from build123d import *

# Parameters (mm, degrees)
F0_W     = 53
F0_H     = 93
F1_DEPTH = 1
F2_W     = 53
F2_H     = 93
F3_DEPTH = 10
F5_DEPTH = 70
F6_W     = 6
F6_H     = 95.9582039332
F6_H_2   = 4.0417960668
F7_DEPTH = 9
F8_DEPTH = 60


with BuildPart() as f1:
    # F0 (on Top) → F1 (new body)
    with BuildSketch(Plane.XY):
        with Locations((-26.5, 46.5)):
            Rectangle(F0_W, F0_H)
    extrude(amount=F1_DEPTH)

    # F2 (on face) → F3 (join)
    with BuildSketch(Plane.XY.offset(1)):
        with Locations((-26.5, 46.5)):
            Rectangle(F2_W, F2_H)
    extrude(amount=-F3_DEPTH)

    # F4 (on face) → F5 (cut)
    with BuildSketch(Plane.YZ):
        Polygon((93, -9), (92.4582039325, -9), (79.0417960675, -9), (78.4996898418, -9), (77.9999999123, -9), (77.4582039325, -9), (64.0417960675, -9), (63.4996898418, -9), (62.9999999123, -9), (62.4582039325, -9), (49.0417960675, -9), (48.4996898418, -9), (47.9999999123, -9), (47.4582039325, -9), (34.0417960675, -9), (33.4996898418, -9), (32.9999999123, -9), (32.4582039318, -9), (19.0417960668, -9), (18.4996898418, -9), (17.9999999123, -9), (17.4582039318, -9), (4.0417960668, -9), (0, -9), (0, -7.7468557283), (-7.4705565355, -7.7468557283), (-7.4705565355, -22.4550403655), (98.083905875, -22.4550403655), (98.083905875, -6.994248211), (93, -6.994248211), align=None)
        with BuildLine():
            Line((79.0417960675, -9), (92.4582039325, -9))
            ThreePointArc((92.4582039325, -9), (92.6770814653, -8.0077412234), (92.7499976369, -6.994248211))
            ThreePointArc((92.7499976369, -6.994248211), (84.7365672438, -0.0737489182), (79.0417960675, -9))
        make_face()
        with BuildLine():
            Line((64.0417960675, -9), (77.4582039325, -9))
            ThreePointArc((77.4582039325, -9), (71.760587075, -0.0733331419), (63.75, -7))
            ThreePointArc((63.75, -7), (63.8233331419, -8.010587075), (64.0417960675, -9))
        make_face()
        with BuildLine():
            Line((34.0417960675, -9), (47.4582039325, -9))
            ThreePointArc((47.4582039325, -9), (40.75, 0), (34.0417960675, -9))
        make_face()
        with BuildLine():
            ThreePointArc((62.4582039325, -9), (62.6766668581, -8.010587075), (62.75, -7))
            ThreePointArc((62.75, -7), (54.739412925, -0.0733331419), (49.0417960675, -9))
            Line((49.0417960675, -9), (62.4582039325, -9))
        make_face()
        with BuildLine():
            ThreePointArc((32.4582039318, -9), (25.7499999993, 0), (19.0417960668, -9))
            Line((19.0417960668, -9), (32.4582039318, -9))
        make_face()
        with BuildLine():
            ThreePointArc((17.4582039318, -9), (11.3890997117, -0.0292359416), (3.7899564275, -7.7468557283))
            ThreePointArc((3.7899564275, -7.7468557283), (3.8872133859, -8.3791881304), (4.0417960668, -9))
            Line((4.0417960668, -9), (17.4582039318, -9))
        make_face()
    extrude(amount=-F5_DEPTH, mode=Mode.SUBTRACT)

    # F6 (on face) → F7 (cut)
    with BuildSketch(Plane(origin=(0, 0, -9), x_dir=(1, 0, 0), z_dir=(0, 0, -1))):
        with Locations((-50, -52.0208980334)):
            Rectangle(F6_W, F6_H)
        with Locations((-50, -2.0208980334)):
            Rectangle(F6_W, F6_H_2)
        with Locations((-3, -2.0208980334)):
            Rectangle(F6_W, F6_H_2)
        with Locations((-3, -52.0208980334)):
            Rectangle(F6_W, F6_H)
    extrude(amount=-F7_DEPTH, mode=Mode.SUBTRACT)

    # F4 (on face) → F8 (cut)
    with BuildSketch(Plane.YZ):
        with BuildLine():
            Line((17.9996898451, -1.9988527525), (17.9999999123, -9))
            Line((17.9999999123, -9), (18.4996898418, -9))
            Line((18.4996898418, -9), (18.4999999113, -6.9988527429))
            Line((18.4999999113, -6.9988527429), (18.4996898418, -1.9988527525))
            ThreePointArc((18.4996898418, -1.9988527525), (18.2496898435, -1.7488527542), (17.9996898451, -1.9988527525))
        make_face()
        with BuildLine():
            Line((32.9996898451, -1.9988527525), (32.9999999123, -9))
            Line((32.9999999123, -9), (33.4996898418, -9))
            Line((33.4996898418, -9), (33.4999999113, -6.9988527429))
            Line((33.4999999113, -6.9988527429), (33.4996898418, -1.9988527525))
            ThreePointArc((33.4996898418, -1.9988527525), (33.2496898435, -1.7488527542), (32.9996898451, -1.9988527525))
        make_face()
        with BuildLine():
            Line((47.9999999123, -9), (48.4996898418, -9))
            Line((48.4996898418, -9), (48.4999999113, -6.9988527429))
            Line((48.4999999113, -6.9988527429), (48.4996898418, -1.9988527525))
            ThreePointArc((48.4996898418, -1.9988527525), (48.2496898435, -1.7488527542), (47.9996898451, -1.9988527525))
            Line((47.9996898451, -1.9988527525), (47.9999999123, -9))
        make_face()
        with BuildLine():
            Line((62.9999113362, -7), (63.4999997335, -7))
            Line((63.4999997335, -7), (63.4999999113, -6.9988527429))
            Line((63.4999999113, -6.9988527429), (63.4996898418, -1.9988527525))
            ThreePointArc((63.4996898418, -1.9988527525), (63.2496898435, -1.7488527542), (62.9996898451, -1.9988527525))
            Line((62.9996898451, -1.9988527525), (62.9999113362, -7))
        make_face()
        with BuildLine():
            Line((77.9999999123, -9), (78.4996898418, -9))
            Line((78.4996898418, -9), (78.4999999113, -6.9988527429))
            Line((78.4999999113, -6.9988527429), (78.4996898418, -1.9988527525))
            ThreePointArc((78.4996898418, -1.9988527525), (78.2496898435, -1.7488527542), (77.9996898451, -1.9988527525))
            Line((77.9996898451, -1.9988527525), (77.9999999123, -9))
        make_face()
        Polygon((63.4996898418, -9), (63.4999997335, -7), (62.9999113362, -7), (62.9999999123, -9), align=None)
    extrude(amount=-F8_DEPTH, mode=Mode.SUBTRACT)


solid = f1.part
Part model, mm, in its own coordinate system. A direction names the side the tool comes from. Give positions to 0.01 mm unless a question says otherwise; leave off trailing zeros. Loops run counter-clockwise (first coordinate to the right, second up) from the corner with the lowest first, then second, coordinate; pieces in that order, holes last.
(1) Band-saw the part on C-C (y = 80). Write the cut outline in (x, z), and give its area (3 significant figures).
Return value:
outline: (-53, 0) - (-47, 0) - (-47, -3.01) - (-6, -3.01) - (-6, 0) - (0, 0) - (0, 1) - (-53, 1) - close
area: 176 mm2
(2) Pin check, flat tips, straight feed: pin 1 (6 mm diameter, centred on y = 80.5, z = -0.5, fed in from +X); pin 2 (1 mm diameter, centred on x = -27.5, y = 58, fed in from -Z); pin 3 (2.5 mm diameter, centred on y = 3.5, z = -2.5, fed in from +X); pin 4 (8 mm diameter, centred on x = -23.5, y = 25, fed in from -Z). Stop position of each tip, or through.
Return value:
pin 1: stops at x = 0
pin 2: stops at z = -0.56
pin 3: stops at x = -6
pin 4: stops at z = -1.86
(3) Pull direction Y, two halves, no side cores. Call faces 1 (the flat face through (-27, 0, -4)), 2 (the flat face through (-6, 33.2, -1.5)), 3 (the cylindrical face through (-26.2, 40.9, 0)): pulls with the +Y half, pulls with the -Y half, needs draft (parallel to the pull), parting line crosses it, or undercut.
Return value:
face 1: pulls with the -Y half
face 2: needs draft
face 3: undercut
(4) Band-saw the part on A-A (y = 66.5). Write the cut outline in (x, z), and give its area (3 significant figures).
Return value:
outline: (-53, 0) - (-47, 0) - (-47, -1.44) - (-6, -1.44) - (-6, 0) - (0, 0) - (0, 1) - (-53, 1) - close
area: 112 mm2
(5) Band-saw the part on B-B (z = -4). Count the separate pieces of the cut face and the enclosed holes in it, and give its area (3 significant figures).
Return value:
separate pieces: 12
enclosed holes: 0
area: 599 mm2
(6) Drill centre lines: line 1 along X through (y, z) = (33, -1.75); line 2 along Z through (x, y) = (-35.5, 10.75); line 3 along Z through (x, y) = (-11.5, 81). Where is each one in solid material? Low to high.
Return value:
line 1: x = -47 to -6
line 2: z = 0 to 1
line 3: z = -1.86 to 1
(7) 3-axis set-ups, long thin cutter, end or side, ignore diameter. For faces 4 (the flat face through (-6, 63.2, -1.5)), 5 (the cylindrical face through (-26.2, 25.9, 0)), 6 (the flat face through (-47, 92, -2)): which of +Z, -Z, +X, -X, +Y, -Y reach the whole face in a straight line?
Return value:
face 4: -Z, +X, +Y, -Y
face 5: +X, -X
face 6: -Z, -X, +Y, -Y
